For this review, take the finished solid that the model builds, in its own axes (mm). Face numbers are marked on the shaded views. Round coordinates to 2 decimals unless told otherwise and drop trailing zeros. Loops run counter-clockwise (first coordinate to the right, second up) from the corner with the lowest first, then second, coordinate; pieces in that order, holes last.
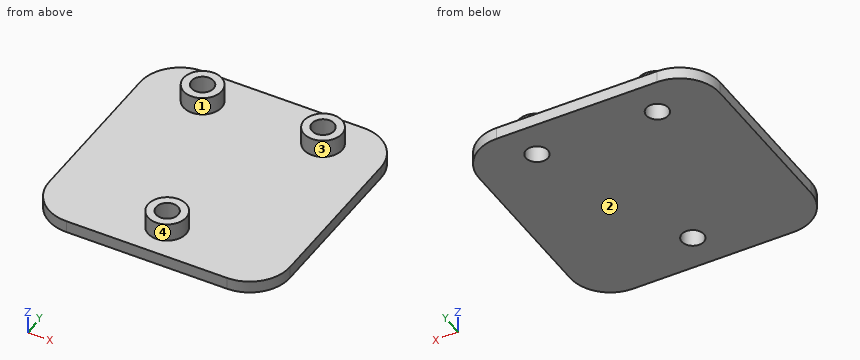
```python
from build123d import *

# Parameters (mm, degrees)
SKETCH1_R           = 2.75
BOSS_EXTRUDE1_DEPTH = 3
SKETCH6_R           = 4.75
SKETCH6_R_2         = 2.75
BOSS_EXTRUDE3_DEPTH = 4.5


with BuildPart() as part:
    # Sketch1 → Boss-Extrude1 (new body)
    with BuildSketch(Plane.XY):
        with BuildLine():
            Line((-20, -30), (20, -30))
            ThreePointArc((20, -30), (27.071067812, -27.071067812), (30, -20))
            Line((30, -20), (30, 20))
            ThreePointArc((30, 20), (27.071067812, 27.071067812), (20, 30))
            Line((20, 30), (-20, 30))
            ThreePointArc((-20, 30), (-27.071067812, 27.071067812), (-30, 20))
            Line((-30, 20), (-30, -20))
            ThreePointArc((-30, -20), (-27.071067812, -27.071067812), (-20, -30))
        make_face()
        with Locations((-15, 21)):
            Circle(SKETCH1_R, mode=Mode.SUBTRACT)
        with Locations((0, -21)):
            Circle(SKETCH1_R, mode=Mode.SUBTRACT)
        with Locations((15, 21)):
            Circle(SKETCH1_R, mode=Mode.SUBTRACT)
    extrude(amount=BOSS_EXTRUDE1_DEPTH)

    # Sketch6 → Boss-Extrude3 (add)
    with BuildSketch(Plane.XY.offset(3)):
        with Locations((-15, 21)):
            Circle(SKETCH6_R)
        with Locations((-15, 21)):
            Circle(SKETCH6_R_2, mode=Mode.SUBTRACT)
        with Locations((0, -21)):
            Circle(SKETCH6_R)
        with Locations((0, -21)):
            Circle(SKETCH6_R_2, mode=Mode.SUBTRACT)
        with Locations((15, 21)):
            Circle(SKETCH6_R)
        with Locations((15, 21)):
            Circle(SKETCH6_R_2, mode=Mode.SUBTRACT)
    extrude(amount=BOSS_EXTRUDE3_DEPTH)


solid = part.part
```
(1) Add section C-C (y = 21). Give the boundary of the cut face in (x, z), plus the area to 3 significant figures.
(2) The part is to be moulded in two halves that separate along X. For the marked faces 1, 2, 3 and 4, say which applies: pulls with the +X half, pulls with the -X half, needs draft (parallel to the pull), parting line crosses it, or undercut.
(3) Add section B-B (x = 15). Give the boundary of the cut face in (y, z), plus the area to 4 significant figures.
(4) Add section A-A (z = 4). Give the boundary of the cut face in (x, y), plus the area to 3 significant figures.
(5) For L1, parallel to Y at x = -15, z = 4.5; L2, parallel to Y at x = 0, z = 3.75; L3, parallel to Z at x = -7, y = -1, list the stretches that pass through material, from the lowest coordinate up.
(6) Insertion check: pin 1 Ø1.5 at (x, y) = (14.5, -17.5) entering from +Z; pin 2 Ø7 at (x, y) = (15, 21) entering from -Z; pin 3 Ø4.5 at (x, y) = (-15, 21) entering from -Z. Each pin has a flat end and moves straight along its axis. Give the tip position at first contact, or say it passes through.
(7) Add section D-D (y = -5.5). Give the boundary of the cut face in (x, z).
Outcome:
1. outline: (-29.95, 0) - (-17.75, 0) - (-17.75, 7.5) - (-19.75, 7.5) - (-19.75, 3) - (-29.95, 3) - close; (-12.25, 0) - (12.25, 0) - (12.25, 7.5) - (10.25, 7.5) - (10.25, 3) - (-10.25, 3) - (-10.25, 7.5) - (-12.25, 7.5) - close; (17.75, 0) - (29.95, 0) - (29.95, 3) - (19.75, 3) - (19.75, 7.5) - (17.75, 7.5) - close
1. area: 183 mm2
2. face 1: undercut
2. face 2: needs draft
2. face 3: undercut
2. face 4: parting line crosses it
3. outline: (-30, 0) - (18.25, 0) - (18.25, 7.5) - (16.25, 7.5) - (16.25, 3) - (-30, 3) - close; (23.75, 0) - (30, 0) - (30, 3) - (25.75, 3) - (25.75, 7.5) - (23.75, 7.5) - close
3. area: 181.5 mm2
4. outline: circle Ø9.5 at (-15, 21); circle Ø9.5 at (0, -21); circle Ø9.5 at (15, 21); hole circle Ø5.5 at (-15, 21); hole circle Ø5.5 at (0, -21); hole circle Ø5.5 at (15, 21)
4. area: 141 mm2
5. L1: y = 16.25 to 18.25, 23.75 to 25.75
5. L2: y = -25.75 to -23.75, -18.25 to -16.25
5. L3: z = 0 to 3
6. pin 1: stops at z = 3
6. pin 2: stops at z = 0
6. pin 3: passes through
7. outline: (-30, 0) - (30, 0) - (30, 3) - (-30, 3) - close
